Can you work these out from the model? Positions are in its coordinate system, mm. A direction names the side the tool comes from. Coordinates: 2 decimals unless noted, no trailing zeros. Order: outer loops, then holes, each group sorted by start corner. A loop starts at its lowest first (then second) coordinate and runs counter-clockwise, first axis right, second up. Notation, with made-up numbers: (-22.75, 25.5) -> (-0.75, 25.5) arc R23 cw to (-0.75, 51.5) -> close; hole circle Ø2 at (5, 17.5). An arc over 180 degrees is marked (long way). Answer as a JSON object with one key per item and string values. Group by question number.
(1) Which directions (+Z, -Z, +X, -X, +Y, -Y) give clear straight access to the entire face, cutting with the end or side of a thin tool? Please do faces 1 (the cylindrical face through (21.73, -1.08, 4.88)), 2 (the conical face through (-6.226, 4.133, -7.199)).
(2) I want a section at A-A, the plane x = 40. List the corners of the cut face in (y, z) for me, plus the area to 3 significant figures.
(3) For pin 1 (2 mm diameter, centred on x = 20, z = -0.5, fed in from +Y); pin 2 (8 mm diameter, centred on x = 33.5, y = -6, fed in from +Z); pin 3 (4 mm diameter, centred on x = -0.5, y = 7, fed in from +Z), each with a flat end and sliding along its axis, tell me the tip position at first contact or that it passes through.
(4) I need wall thicknesses on line 1 (X direction, y = 0, z = -6); line 2 (X direction, y = 3.5, z = -3.5); line 3 (Z direction, x = 17.5, y = -4). Which ranges of each line are inside material? Lowest first, please.
Autodesk Inventor part; units mm, degrees
ref_plane "Work Plane1" through (1.525, 0, 0) normal (0, 0, 1) x (1, 0, 0)
ref_plane "YZ Plane" through (0, 0, 0) normal (1, 0, 0) x (0, 1, 0)
ref_plane "XZ Plane" through (0, 0, 0) normal (0, 1, 0) x (-1, 0, 0)
sketch "Sketch1" plane through (0, 0, 0) normal (0, 0, 1) x (1, 0, 0)
  line L0 (0, 7.315) -> (0, 5)
  line L1 (19, 5) -> (45, 5)
  line L2 (45, 5) -> (45, 0)
  line L3 (45, 0) -> (-0.6001, 0)
  line L4 (-9.7201, 0) -> (54.12, 0)
  line L5 (-0.6001, 0) -> (-0.6001, 7.315)
  line L6 (-0.6001, 7.315) -> (0, 7.315)
  line L7 (19, 5) -> (18.0797, 5)
  line L8 (18.0797, 5) -> (0, 5)
  line L9 (0, -1.463) -> (0, 8.778)
  dimension "d0" = 45
  dimension "d1" = 26
  dimension "d2" = 10
  dimension "d9" = 0.6001
  dimension "d10" = 14.63
  dimension "d13" = 0.9203
  dimension "d14" = 10
revolve "Body" add sketch "Sketch1" angle 360 about axis through (45, 0, 0) along (-1, 0, 0)
sketch "Sketch2" plane through (-0.6001, 0, 0) normal (-1, 0, 0) x (0, 0, 1)
  line L0 (0, 9.2376) -> (8, 4.6188)
  line L1 (8, 4.6188) -> (8, -4.6188)
  line L2 (8, -4.6188) -> (0, -9.2376)
  line L3 (0, -9.2376) -> (-8, -4.6188)
  line L4 (-8, -4.6188) -> (-8, 4.6188)
  line L5 (-8, 4.6188) -> (0, 9.2376)
  point P0 (0, 0)
  point P1 (0, 0)
  dimension "d11" = 16
extrude "Head" add sketch "Sketch2" along normal blind 5.8
sketch "Sketch4" plane through (0, 0, 0) normal (0, 0, 1) x (1, 0, 0)
  line L0 (-6.4001, 8) -> (-6.4001, 9.2376)
  line L1 (-6.4001, 9.2376) -> (-5.6856, 9.2376)
  line L2 (-5.6856, 9.2376) -> (-6.4001, 8)
  line L3 (-7.5601, 0) -> (0.5599, 0)
  line L4 (-0.6001, 9.2376) -> (-6.4001, 9.2376)
  line L5 (-6.4001, 4.6188) -> (-6.4001, 9.2376)
  dimension "d5" = 30
  dimension "d19" = 16
revolve "Chamfer1" cut sketch "Sketch4" angle 360 about axis through (-10, 0, 0) along (1, 0, 0)
thread "Thread"
chamfer "Chamfer2" distance 0.9202 distance2 0.9203 1 edges at (45, -5, 0) measured on face at (45, 1.2281, 0.495)
ref_plane "Work Plane1" through (1.525, 0, 0) normal (0, 0, 1) x (1, 0, 0)
equation "\"d0\" = NLG"
equation "\"d1\" = GEL"
equation "\"d2\" = GD"
equation "\"d10\" = SD2"
equation "\"d14\" = BDM"
equation "\"d11\" = SW"
equation "\"d3\" = KOH - SD"
equation "\"d5\" = ANG1"
equation "\"d19\" = SW0"
equation "\"d15\" = GEL"
equation "\"d6\" = -0.5 * SPD + 0.5 * GD"
equation "\"NLG\" = 45"
equation "\"GD\" = NND"
equation "\"BDM\" = NND"
equation "\"KOH\" = 6.4"
equation "\"GEL\" = 26"
equation "\"SW\" = 16"
equation "\"SW0\" = SW"
equation "\"SPD\" = NND - 1.2269 * PTC"
equation "\"SD2\" = 14.63"
equation "\"SD\" = 0.6"
equation "\"ANG1\" = 30deg"
equation "\"GAL\" = 0.61345 * PTC"
equation "\"GUL\" = 0.61345 * PTC"
equation "\"RR\" = 0.4"
equation "\"GD1\" = THREADDIA - 1.2269 * PTC"
equation "\"SDH\" = SD2"
equation "\"TOA\" = 30deg"
equation "\"PTC\" = 1.5"
equation "\"E0\" = 1.155 * SW"
properties part number "ISO 4014 - M10 x 45" material "Stainless Steel, 440C"
Computed values:
{
 "1": {"face 1": "+X", "face 2": "-Z, -X, +Y"},
 "2": {"outline": "circle Ø10 at (0, 0)", "area": "78.5 mm2"},
 "3": {"pin 1": "stops at y = 5", "pin 2": "stops at z = 4.58", "pin 3": "stops at z = 7.34"},
 "4": {"line 1": "x = -6.4 to 0", "line 2": "x = -6.4 to 44.13", "line 3": "z = -3 to 3"}
}
